For this review, take the finished solid that the model builds, in its own axes (mm). Face numbers are marked on the shaded views. A direction names the side the tool comes from. Coordinates: 2 decimals unless noted, no trailing zeros. Write each loop counter-clockwise with the first axis right and the second up, starting at its lowest first coordinate (ties: lowest second). Pieces come first, ordered by that corner, then holes.
```python
from build123d import *

# Parameters (mm, degrees)
SKETCH_1_W          = 7.5
SKETCH_1_H          = 6
EXTRUDE_1_DEPTH     = 7
SHELL_1_T           = -1
CUT_EXTRUDE_1_REACH = 8
SKETCH_2_W          = 4
SKETCH_2_H          = 4
EXTRUDE_START       = -7
SKETCH_3_W          = 0.6
SKETCH_3_H          = 0.6
EXTRUDE_2_DEPTH     = 10


with BuildPart() as part:
    # 草图1 → 凸台-拉伸1 (new body)
    with BuildSketch(Plane(origin=(0, 0, 0), x_dir=(1, 0, 0), z_dir=(0, 1, 0))):
        Rectangle(SKETCH_1_W, SKETCH_1_H)
    extrude(amount=EXTRUDE_1_DEPTH)

    # 抽壳1
    shell_1_openings = [part.faces().sort_by_distance(p)[0] for p in [
        (0, 7, 0),
    ]]
    offset(amount=SHELL_1_T, openings=shell_1_openings, kind=Kind.INTERSECTION)

    # 草图2 → 切除-拉伸1 (cut, up to next)
    with BuildSketch(Plane.XY.offset(3), mode=Mode.PRIVATE) as cut_extrude_1_sk1:
        with Locations((0, 5)):
            Rectangle(SKETCH_2_W, SKETCH_2_H)
    cut_extrude_1_tool1 = extrude(cut_extrude_1_sk1.sketch, amount=-CUT_EXTRUDE_1_REACH, mode=Mode.PRIVATE) & part.part
    add(cut_extrude_1_tool1.solids().sort_by_distance((0, 5, 3))[0], mode=Mode.SUBTRACT)

    # 草图3 → 凸台-拉伸2 (add)
    with BuildSketch(Plane.XZ.offset(EXTRUDE_START)):
        with Locations((-1.2, 0.3)):
            Rectangle(SKETCH_3_W, SKETCH_3_H)
        with Locations((1.2, 0.3)):
            Rectangle(SKETCH_3_W, SKETCH_3_H)
    extrude(amount=EXTRUDE_2_DEPTH)


solid = part.part
```
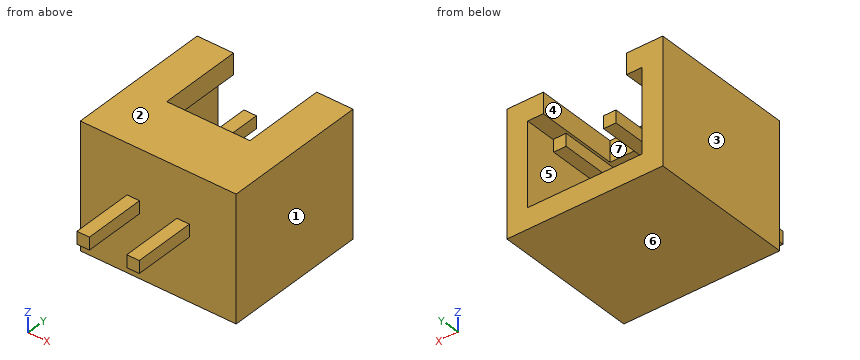
Q1. For probe 1 along Z at (x, y) = (2.25, 3.5); probe 2 along X at (y, z) = (4.5, 1.7); probe 3 along Z at (x, y) = (-1, 6.5), list the stretches that pass through material, from the lowest coordinate up.
Ans:
probe 1: z = -3 to -2, 2 to 3
probe 2: x = -3.75 to -2.75, 2.75 to 3.75
probe 3: z = -3 to -2, 0 to 0.6
Q2. Add section A-A (y = 4). State the section outline as (x, z) points, then the cut area to 3 significant figures.
Ans:
outline: (-3.75, -3) - (3.75, -3) - (3.75, 3) - (2, 3) - (2, 2) - (2.75, 2) - (2.75, -2) - (-2.75, -2) - (-2.75, 2) - (-2, 2) - (-2, 3) - (-3.75, 3) - close; (-1.5, 0) - (-0.9, 0) - (-0.9, 0.6) - (-1.5, 0.6) - close; (0.9, 0) - (1.5, 0) - (1.5, 0.6) - (0.9, 0.6) - close
area: 19.7 mm2
Q3. Add section C-C (z = 0.35). State the section outline as (x, y) points.
Ans:
outline: (-3.75, 0) - (-1.5, 0) - (-1.5, -3) - (-0.9, -3) - (-0.9, 0) - (0.9, 0) - (0.9, -3) - (1.5, -3) - (1.5, 0) - (3.75, 0) - (3.75, 7) - (2.75, 7) - (2.75, 1) - (1.5, 1) - (1.5, 7) - (0.9, 7) - (0.9, 1) - (-0.9, 1) - (-0.9, 7) - (-1.5, 7) - (-1.5, 1) - (-2.75, 1) - (-2.75, 7) - (-3.75, 7) - close
Q4. Add section B-B (x = -2.25). State the section outline as (y, z) points, then the cut area to 3 significant figures.
Ans:
outline: (0, -3) - (7, -3) - (7, -2) - (1, -2) - (1, 2) - (7, 2) - (7, 3) - (0, 3) - close
area: 18.0 mm2
Q5. Clearance check with flat-ended pins moving along their axes: pin 1 Ø0.7 at (x, y) = (-1.5, 4.5) entering from +Z; pin 2 Ø1.2 at (x, z) = (-1.5, -1) entering from +Y; pin 3 Ø0.8 at (x, z) = (1, 2.5) entering from +Y. State where each tip first meets the part, or that it passes through.
Ans:
pin 1: stops at z = 0.6
pin 2: stops at y = 1
pin 3: stops at y = 3
Q6. Draft analysis for pull direction X (two halves, no side actions). For the marked faces 1, 2, 3 and 4, state which applies: +X half, -X half, draft (parallel to the pull), parting line (faces both ways), or undercut.
Ans:
face 1: +X half
face 2: draft
face 3: -X half
face 4: undercut
Q7. Tool access review of the marked faces 5, 6 and 7: name each direction out of +Z, -Z, +X, -X, +Y, -Y from which nothing blocks a thin tool from reaching the whole face with its end or side.
Ans:
face 5: +Y
face 6: -Z, +X, -X, +Y, -Y
face 7: +Z, +Y
Q8. Add section D-D (z = -0.6). State the section outline as (x, y) points, then the cut area to 3 significant figures.
Ans:
outline: (-3.75, 0) - (3.75, 0) - (3.75, 7) - (2.75, 7) - (2.75, 1) - (-2.75, 1) - (-2.75, 7) - (-3.75, 7) - close
area: 19.5 mm2
